```python
from build123d import *

# Parameters (mm, degrees)
SKETCH1_W               = 25.4
SKETCH1_H               = 25.4
BOSS_EXTRUDE1_DEPTH     = 57.15
CUT_EXTRUDE1_DEPTH      = 64.816710194
CUT_EXTRUDE1_DEPTH_BACK = 64.816710194
SKETCH2_R               = 2.0701
SKETCH4_R               = 4.7625
CUT_EXTRUDE2_DEPTH      = 25.4
CHAMFER1_SIZE           = 1.27
FILLET1_R               = 6.35
FILLET2_R               = 6.35


with BuildPart() as part:
    # Sketch1 → Boss-Extrude1 (new body)
    with BuildSketch(Plane.XY):
        Rectangle(SKETCH1_W, SKETCH1_H)
    extrude(amount=BOSS_EXTRUDE1_DEPTH)

    # Sketch2 → Cut-Extrude1 (cut, two sides: drawn at the far end of the back side and taken through both)
    with BuildSketch(Plane(origin=(0, 12.7, 0), x_dir=(1, 0, 0), z_dir=(0, 1, 0)).offset(-CUT_EXTRUDE1_DEPTH_BACK)):
        with BuildLine():
            Line((-12.7, 0), (-12.7, -29.5402))
            Line((-12.7, -29.5402), (-5.027345066, -3.749481199))
            ThreePointArc((-5.027345066, -3.749481199), (-3.135793664, -1.040593833), (7e-09, 0))
            Line((7e-09, 0), (-12.7, 0))
        make_face()
        with BuildLine():
            Line((5.027345066, -3.749481199), (12.7, -29.5402))
            Line((12.7, -29.5402), (12.7, 0))
            Line((12.7, 0), (7e-09, 0))
            ThreePointArc((7e-09, 0), (3.135793669, -1.040593837), (5.027345066, -3.749481199))
        make_face()
        with Locations(Location((0, -5.2451, 0), (0, 0, 180))):
            Circle(SKETCH2_R)
        with Locations(Location((0, -24.2951, 0), (0, 0, 180))):
            Circle(SKETCH2_R)
    extrude(amount=CUT_EXTRUDE1_DEPTH + CUT_EXTRUDE1_DEPTH_BACK, mode=Mode.SUBTRACT)

    # Sketch4 → Cut-Extrude2 (cut)
    with BuildSketch(Plane.XY.offset(57.15)):
        Circle(SKETCH4_R)
    extrude(amount=-CUT_EXTRUDE2_DEPTH, mode=Mode.SUBTRACT)

    # Chamfer1
    chamfer1_edges = [part.edges().sort_by_distance(p)[0] for p in [
        (-4.7625, 0, 57.15),
    ]]
    chamfer(chamfer1_edges, length=CHAMFER1_SIZE)

    # Fillet1
    fillet1_edges = [part.edges().sort_by_distance(p)[0] for p in [
        (12.7, 0, 57.15),
        (-12.7, 0, 57.15),
        (0, -12.7, 57.15),
        (12.7, -12.7, 43.3451),
        (-12.7, -12.7, 43.3451),
    ]]
    fillet(fillet1_edges, radius=FILLET1_R)

    # Fillet2
    fillet2_edges = [part.edges().sort_by_distance(p)[0] for p in [
        (-12.7, 12.7, 40.1701),
        (12.7, 12.7, 40.1701),
        (0, 12.7, 57.15),
        (10.840128061, 12.7, 55.290128061),
        (-10.840128061, 12.7, 55.290128061),
    ]]
    fillet(fillet2_edges, radius=FILLET2_R)


solid = part.part
```
Work out the finished part from the listing and answer in its coordinate system (mm). A direction names the side the tool comes from. Round coordinates to 2 decimals unless told otherwise and drop trailing zeros. Loops run counter-clockwise (first coordinate to the right, second up) from the corner with the lowest first, then second, coordinate; pieces in that order, holes last. Notation, with made-up numbers: M 35.5,22.5 L 77.5,22.5 A26 ccw 77.5,54.5 Z; hole C 53.25,-36.5 d2. An arc over 180 degrees is marked long. One line per question, with ' | ' between items.
Q1. The mould has two halves that part along X. Classify faces 3 (the cylindrical face through (-3.78, -2.9, 43.98)), 4 (the flat face through (-8.92, -0.18, 16.83)), 5 (the cylindrical face through (9.935, -11.591, 34.53)): +X half, -X half, draft (parallel to the pull), parting line (faces both ways), or undercut.
Conclusion:
face 3: undercut | face 4: -X half | face 5: +X half
Q2. Find section C-C, the plane z = 23.5. Give the vertices of the cut face in (x, y).
Conclusion:
outline: M -10.9,-10.78 A6.35 ccw -6.35,-12.7 L -1.91,-12.7 L -1.91,12.7 L -6.35,12.7 A6.35 ccw -10.9,10.78 Z; M 1.91,-12.7 L 6.35,-12.7 A6.35 ccw 10.9,-10.78 L 10.9,10.78 A6.35 ccw 6.35,12.7 L 1.91,12.7 Z
Q3. A tool of negligible diameter and unlimited length cuts with its end or side. For faces 1 (the flat face through (0, 0, 31.75)), 2 (the flat face through (3, 12.7, 25)), from which of +Z, -Z, +X, -X, +Y, -Y can it reach the whole face along a straight path? Write none if from no direction.
Conclusion:
face 1: +Z | face 2: +Z, -Z, +X, -X, +Y
Q4. Consider line 1 along Z through (x, y) = (-1.75, 11.5); line 2 along Y through (x, z) = (0, 49.25); line 3 along X through (y, z) = (10.5, 25). Determine where each line is inside the solid, lowest interval first. Write a range as from..to.
Conclusion:
line 1: z = 0.3..4.14, 6.35..23.19, 25.4..54.51 | line 2: y = -12.7..-4.76, 4.76..12.7 | line 3: x = -11.16..-1.95, 1.95..11.16
Q5. Find section B-B, the plane y = -7.75. Give the vertices of the cut face in (x, z), then the cut area to 3 significant figures.
Conclusion:
outline: M -12.54,29.01 L -5.03,3.75 A5.25 ccw 5.03,3.75 L 12.54,29.01 L 12.54,50.8 A6.19 ccw 6.35,56.99 L -6.35,56.99 A6.19 ccw -12.54,50.8 Z; hole C 0,5.25 d4.14; hole C 0,24.3 d4.14 | area: 1,130 mm2
Q6. Find section D-D, the plane y = -11. Give the vertices of the cut face in (x, z), then the cut area to 3 significant figures.
Conclusion:
outline: M -10.67,22.73 L -5.03,3.75 A5.25 ccw 5.03,3.75 L 10.67,22.73 L 10.67,50.8 A4.32 ccw 6.35,55.12 L -6.35,55.12 A4.32 ccw -10.67,50.8 Z; hole C 0,5.25 d4.14; hole C 0,24.3 d4.14 | area: 982 mm2
Q7. Each of these flat-tipped pins is pushed along its axis until it touches: pin 1 Ø5 at (y, z) = (2.5, 7.5) entering from -X; pin 2 Ø2 at (x, y) = (-4.5, -3.5) entering from -Z; pin 3 Ø3 at (x, y) = (3, 8) entering from -Z. Where does it stop, or does it pass through?
Conclusion:
pin 1: stops at x = -6.89 | pin 2: stops at z = 1.34 | pin 3: stops at z = 0.22
